Autodesk Inventor part; units mm, degrees
ref_plane "YZ Plane" through (0, 0, 0) normal (1, 0, 0) x (0, 1, 0)
ref_plane "XZ Plane" through (0, 0, 0) normal (0, 1, 0) x (-1, 0, 0)
ref_plane "XY Plane" through (0, 0, 0) normal (0, 0, 1) x (1, 0, 0)
sketch "Szkic1" plane through (0, 0, 0) normal (1, 0, 0) x (0, 1, 0)
  line L0 (10, 0) -> (130, 0)
  line L1 (130, 0) -> (130, 20)
  line L2 (130, 20) -> (10, 20)
  line L3 (0, 10) -> (0, 10)
  arc A0 (0, 10) -> (10, 0) centre (10, 10) ccw
  arc A1 (10, 20) -> (0, 10) centre (10, 10) ccw
  point P0 (0, 0)
  point P1 (0, 20)
  dimension "d0" = 20
  dimension "d2" = 10
  dimension "d5" = 120
extrude "Wyciągnięcie proste1" add sketch "Szkic1" along normal blind 3
sketch "Szkic2" plane through (3, 0, 0) normal (1, 0, 0) x (0, 0, -1)
  arc A0 (-20, 10) -> (0, 10) centre (-10, 10) ccw
  point P0 (0, 0)
sketch "Szkic3" plane through (3, 0, 0) normal (1, 0, 0) x (0, 0, -1)
  point P0 (0, 0)
  point P1 (-10, 32)
  dimension "d6" = 32
hole "Otwór1" at (3, 32, 10) direction (-1, 0, 0) diameter 3.2 end through all
properties material "Drewno (wiśnia)"
Could you check a few things on this model? Use its own coordinates, in mm. Give positions to 0.01 mm unless a question says otherwise; leave off trailing zeros. Order: outer loops, then holes, each group sorted by start corner. A loop starts at its lowest first (then second) coordinate and runs counter-clockwise, first axis right, second up.
1. Suppose I cut it at B-B (z = 10). Write out the boundary of the cut face in (x, y).
Answers below:
outline: (0, 0) - (3, 0) - (3, 30.4) - (0, 30.4) - close; (0, 33.6) - (3, 33.6) - (3, 130) - (0, 130) - close
2. I need wall thicknesses on L1, parallel to Y at x = 1.25, z = 10; L2, parallel to Z at x = 2.4, y = 32; L3, parallel to Y at x = 0.2, z = 12. Which ranges of each line are inside material? Lowest first, please.
Answers below:
L1: y = 0 to 30.4, 33.6 to 130
L2: z = 0 to 8.4, 11.6 to 20
L3: y = 0.2 to 130
3. Suppose I cut it at A-A (y = 32). Write out the boundary of the cut face in (x, z), plus the area to 3 significant figures.
Answers below:
outline: (0, 0) - (3, 0) - (3, 8.4) - (0, 8.4) - close; (0, 11.6) - (3, 11.6) - (3, 20) - (0, 20) - close
area: 50.4 mm2
4. Suppose I cut it at C-C (x = 1.25). Write out the boundary of the cut face in (y, z), plus the area to 3 significant figures.
Answers below:
outline: (10, 0) - (130, 0) - (130, 20) - (10, 20) arc R10 ccw to start; hole circle Ø3.2 at (32, 10)
area: 2,550 mm2
5. Suppose I cut it at D-D (z = 18.25). Write out the boundary of the cut face in (x, y), plus the area to 3 significant figures.
Answers below:
outline: (0, 4.35) - (3, 4.35) - (3, 130) - (0, 130) - close
area: 377 mm2
6. Thinking about a two-plate mould opening in Y: for faces 1 (the flat face through (3, 64, 10)), 2 (the cylindrical face through (1, 0, 10)), 3 (the cylindrical face through (1.48, 32.97, 11.27)), which applies, +Y half, -Y half, draft (parallel to the pull), parting line (faces both ways), or undercut?
Answers below:
face 1: draft
face 2: -Y half
face 3: undercut
